Read the model definition and answer for the solid it produces. Units are mm, in the model's axes. A direction names the side the tool comes from. Round coordinates to 2 decimals unless told otherwise and drop trailing zeros. Write each loop counter-clockwise with the first axis right and the second up, starting at its lowest first coordinate (ties: lowest second). Pieces come first, ordered by that corner, then holes.
Autodesk Inventor part; units mm, degrees
ref_plane "YZ Plane" through (0, 0, 0) normal (1, 0, 0) x (0, 1, 0)
ref_plane "XZ Plane" through (0, 0, 0) normal (0, 1, 0) x (-1, 0, 0)
ref_plane "XY Plane" through (0, 0, 0) normal (0, 0, 1) x (1, 0, 0)
sketch "Esboço1" plane through (0, 0, 0) normal (0, 1, 0) x (-1, 0, 0)
  line L0 (-10, 10) -> (10, 10) construction
  line L1 (10, 10) -> (10, -10) construction
  line L2 (10, -10) -> (-10, -10) construction
  line L3 (-10, -10) -> (-10, 10) construction
  line L4 (-10, 10) -> (10, -10) construction
  line L5 (10, 10) -> (-10, -10) construction
  line L6 (0, -4.5) -> (3.1, -4.5)
  line L7 (0, -10) -> (0, 10) construction
  line L8 (5.8739, -7.1527) -> (3.4597, -4.6527)
  arc A0 (3.4597, -4.6527) -> (3.1, -4.5) centre (3.1, -5) ccw
  line L9 (5.5142, -8) -> (3.1, -8)
  arc A1 (5.5142, -8) -> (5.8739, -7.1527) centre (5.5142, -7.5) ccw
  line L10 (3.1, -9.5) -> (3.1, -8)
  line L11 (3.6, -9.5) -> (3.1, -9.5)
  line L12 (3.6, -10) -> (3.6, -9.5)
  line L13 (10, -10) -> (3.6, -10) construction
  line L14 (10, -10) -> (0, -10) construction
  line L15 (10, -10) -> (10, -3.6) construction
  line L16 (9.5, -3.1) -> (8, -3.1)
  line L17 (9.5, -3.1) -> (9.5, -3.6)
  line L18 (9.5, -3.6) -> (10, -3.6)
  line L19 (8, -3.1) -> (8, -5.5142)
  line L20 (7.1527, -5.8739) -> (4.6527, -3.4597)
  line L21 (4.5, 0) -> (4.5, -3.1)
  arc A2 (4.5, -3.1) -> (4.6527, -3.4597) centre (5, -3.1) ccw
  line L22 (10, 0) -> (0, 0) construction
  line L23 (4.5, 0) -> (2.5, 0)
  line L24 (0, -4.5) -> (0, -2.5)
  arc A3 (7.1527, -5.8739) -> (8, -5.5142) centre (7.5, -5.5142) ccw
  arc A4 (0, -2.5) -> (2.5, 0) centre (0, 0) ccw
  arc A5 (9.5, -10) -> (10, -9.5) centre (9.5, -9.5) ccw
  line L25 (9.5, -10) -> (3.6, -10)
  line L26 (10, -9.5) -> (10, -3.6)
  point P0 (3.5, 0)
  dimension "d0" = 20
  dimension "d5" = 0.5
  dimension "d6" = 1
  dimension "d7" = 0.5
  dimension "d8" = 2
  dimension "d10" = 6.9
  dimension "d12" = 3.1
  dimension "d15" = 2.5
  dimension "d16" = 2
extrude "Extrusão1" add sketch "Esboço1" along normal mid plane 150
mirror "Espelhar1" about plane through (0, 0, 0) normal (1, 0, 0) of "Extrusão1"
mirror "Espelhar2" about plane through (0, 0, 0) normal (0, 0, 1) of "Extrusão1", "Espelhar1"
equation "\"Raio_vergadura\" = Espessura"
equation "\"Largura_alívio_de_vergadura\" = Espessura"
equation "\"Profundidade_alívio_de_vergadura\" = 0.5 * Espessura"
equation "\"Tamanho_alívio_de_dobra\" = 4 * Espessura"
equation "\"Remanescente_mínimo\" = 2 * Espessura"
equation "\"Raiodetransição\" = Raio_vergadura"
equation "\"Tamanho_de_raio_de_Jacobi\" = Raio_vergadura"
equation "\"TamanhoFolga\" = Espessura"
Q1. Straight lines are drawn through the part: probe 1 along X at (y, z) = (-54, 7.5); probe 2 along X at (y, z) = (44.5, -3.5); probe 3 along X at (y, z) = (-38.5, 0). For each, find the intervals that lie inside material, in ascending order.
Verdict:
probe 1: x = -10 to -6.01, 6.01 to 10
probe 2: x = -9.5 to -8, -4.69 to 4.69, 8 to 9.5
probe 3: x = -4.5 to -2.5, 2.5 to 4.5
Q2. Section A-A (z = 0) is taken. Determine the outline of the cut face in (x, y), then the cut area to 3 significant figures.
Verdict:
outline: (-4.5, -75) - (-2.5, -75) - (-2.5, 75) - (-4.5, 75) - close; (2.5, -75) - (4.5, -75) - (4.5, 75) - (2.5, 75) - close
area: 600 mm2
Q3. Determine the mould class of faces 4 (the flat face through (0, -1, 4.5)), 5 (the flat face through (7, -1, -10)), 6 (the flat face through (-4.684, -1.05, -5.92)) for opening direction Z: pulls with the +Z half, pulls with the -Z half, needs draft (parallel to the pull), parting line crosses it, or undercut.
Verdict:
face 4: pulls with the +Z half
face 5: pulls with the -Z half
face 6: undercut
Q4. Flat-ended cylindrical pins translate along their axes: pin 1 Ø3 at (x, y) = (-1.5, -34) entering from +Z; pin 2 Ø0.6 at (y, z) = (-35.5, -3.5) entering from -X. Find the tip coordinate at first contact, or state that the pin passes through.
Verdict:
pin 1: stops at z = 4.5
pin 2: stops at x = -10
Q5. Which of the six approach directions +Z, -Z, +X, -X, +Y, -Y give full straight-line access (tool end or side, diameter ignored) to faces 1 (the flat face through (4.5, -1, 0)), 2 (the flat face through (-7, -1, 10)), 3 (the flat face through (-5.92, -1.05, -4.684))?
Verdict:
face 1: +X, +Y, -Y
face 2: +Z, +X, -X, +Y, -Y
face 3: +Y, -Y
